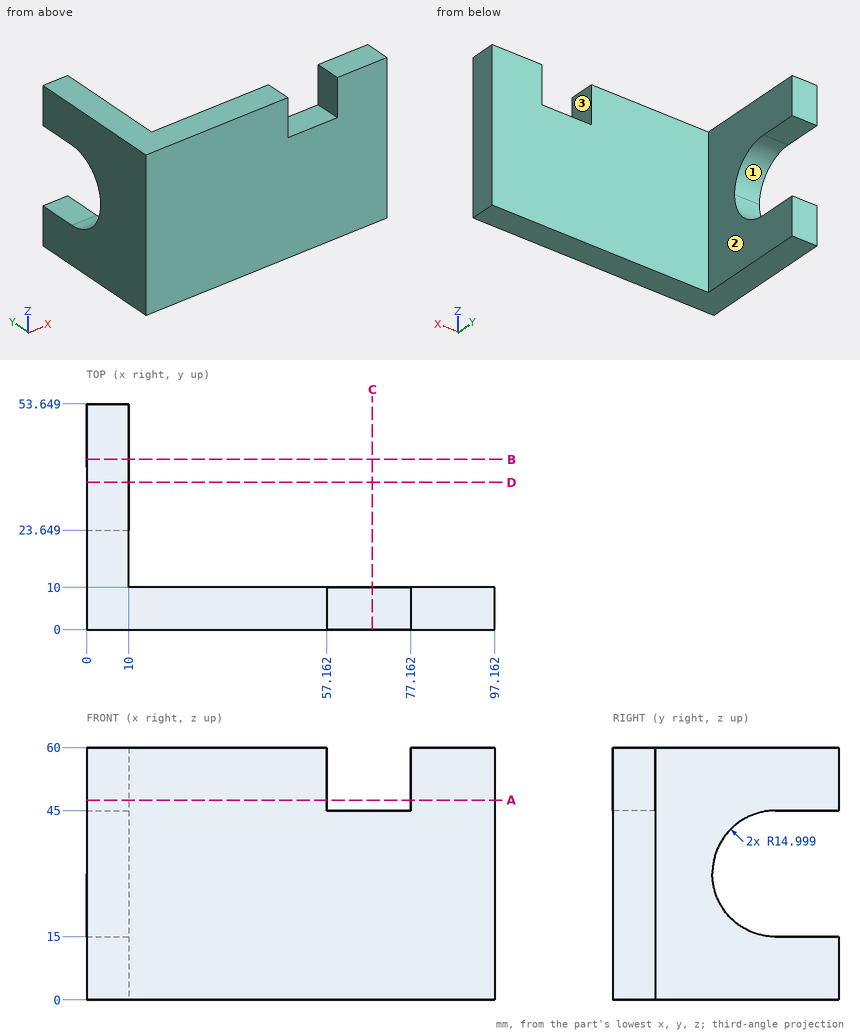
Job drawing, mm, ordinate dimensions from the low corner. One solid piece. A direction names the side the tool comes from. Coordinates: 2 decimals unless noted, no trailing zeros. Order: outer loops, then holes, each group sorted by start corner. A loop starts at its lowest first (then second) coordinate and runs counter-clockwise, first axis right, second up. Notation, with made-up numbers: (39, 19.25) - (75, 19.25) arc R9 ccw to (75, 33.25) - close; hole circle Ø3 at (-37, -5). An arc over 180 degrees is marked (long way). Use CSV: the item, a comma, the result in double quotes.
Item 1: Saw through at A-A on z = 47.5. Give the cut face in (x, y).
Solved:
outline,"(0, 0) - (57.16, 0) - (57.16, 10) - (10, 10) - (10, 53.65) - (0, 53.65) - close; (77.16, 0) - (97.16, 0) - (97.16, 10) - (77.16, 10) - close"
Item 2: Saw through at B-B on y = 40.5. Give the cut face in (x, z).
Solved:
outline,"(0, 0) - (10, 0) - (10, 15) - (0, 15) - close; (0, 45) - (10, 45) - (10, 60) - (0, 60) - close"
Item 3: Saw through at D-D on y = 35. Give the cut face in (x, z), and give its area (3 significant figures).
Solved:
outline,"(0, 0) - (10, 0) - (10, 15.45) - (0, 15.45) - close; (0, 44.55) - (10, 44.55) - (10, 60) - (0, 60) - close"
area,"309 mm²"
Item 4: 3-axis set-ups, long thin cutter, end or side, ignore diameter. For the marked faces 1, 2 and 3: which of +Z, -Z, +X, -X, +Y, -Y reach the whole face in a straight line?
Solved:
face 1,"+X, -X, +Y"
face 2,"+Z, -Z, +X, +Y"
face 3,"+Z, +Y, -Y"
Item 5: Drop flat-ended pins along their axis: P1, Ø10, axis at y = 25.5, z = 28.5, coming from the +X side; P2, Ø3, axis at x = 66, y = 3, coming from the +Z side. Give the stop position or say it passes through.
Solved:
P1,"stops at x = 10"
P2,"stops at z = 45"
Item 6: Saw through at C-C on x = 68. Give the cut face in (y, z), and give its area (3 significant figures).
Solved:
outline,"(0, 0) - (10, 0) - (10, 45) - (0, 45) - close"
area,"450 mm²"
Item 7: Probe probe 1 along X at (y, z) = (10.5, 14.5); probe 2 along Z at (x, y) = (6.5, 33) (1 decimal). List the from-to ranges inside material, lowest first.
Solved:
probe 1,"x = 0 to 10"
probe 2,"z = 0 to 16.1, 43.9 to 60"
